from build123d import *

# Parameters (mm, degrees)
CUT_EXTRUDE1_DEPTH     = 5
CUT_EXTRUDE3_DEPTH     = 45
SKETCH8_R              = 40
CUT_EXTRUDE4_DEPTH     = 32
FILLET1_R              = 7
CUT_REVOLVE1_START     = 17
CUT_REVOLVE1_DEPTH     = 30.5
SKETCH18_W             = 13
SKETCH18_H             = 8
CUT_EXTRUDE13_DEPTH    = 5
SKETCH20_W             = 84
SKETCH20_H             = 7
CUT_EXTRUDE15_DEPTH    = 5
SKETCH19_R             = 1.5
CUT_EXTRUDE14_DEPTH    = 12
FILLET3_R              = 4
SKETCH21_W             = 16
SKETCH21_H             = 5
CUT_EXTRUDE16_DEPTH    = 5
CIRPATTERN1_COUNT      = 4
SKETCH22_W             = 5
SKETCH22_H             = 12
BOSS_EXTRUDE1_DEPTH    = 1.5
SKETCH23_W             = 5
SKETCH23_H             = 4.4
SKETCH23_H_2           = 4
BOSS_EXTRUDE2_DEPTH    = 17
SKETCH24_W             = 2
SKETCH24_H             = 3
BOSS_EXTRUDE3_DEPTH    = 2
CIRPATTERN2_COUNT      = 5
CUT_REVOLVE2_START     = 17
CUT_REVOLVE2_DEPTH     = 30.5
SKETCH29_W             = 16.2
SKETCH29_H             = 11.2
SKETCH29_W_2           = 13
SKETCH29_H_2           = 8
BOSS_EXTRUDE4_DEPTH    = 20
CUT_EXTRUDE18_DEPTH    = 12
SKETCH34_R             = 2.3
BOSS_EXTRUDE5_DEPTH    = 3.5
BOSS_EXTRUDE6_START    = 3.5
SKETCH35_R             = 2.3
BOSS_EXTRUDE6_DEPTH    = 3.5
SKETCH36_W             = 2
SKETCH36_H             = 2
BOSS_EXTRUDE7_DEPTH    = 5
SKETCH37_W             = 2
SKETCH37_H             = 2
BOSS_EXTRUDE8_DEPTH    = 12.5
SKETCH40_W             = 2
SKETCH40_H             = 2
BOSS_EXTRUDE9_DEPTH    = 5
INTERSECT7_START       = -43
INTERSECT7_OUTLINE_W   = 16.2
INTERSECT7_OUTLINE_H   = 20
INTERSECT7_OUTLINE_R   = 2.3
INTERSECT7_DEPTH       = 86
INTERSECT7_START_2     = -35.6
INTERSECT7_2_OUTLINE_W = 16.2
INTERSECT7_2_OUTLINE_H = 20
INTERSECT7_2_OUTLINE_R = 2.3
INTERSECT7_2_DEPTH     = 37.6


with BuildPart() as part:
    # Sketch1 → Revolve1 (revolve)
    with BuildSketch(Plane.XY, mode=Mode.PRIVATE) as revolve1_sk:
        with BuildLine():
            Line((37, 55), (0, 55))
            Line((0, 55), (0, 11.5))
            Line((0, 11.5), (22.5, 11.5))
            Line((22.5, 11.5), (22.5, 0))
            Line((22.5, 0), (25, 0))
            Line((25, 0), (25, 11.5))
            Line((25, 11.5), (42, 11.5))
            Line((42, 11.5), (42, 50))
            ThreePointArc((42, 50), (40.535533906, 53.535533906), (37, 55))
        make_face()
    revolve(revolve1_sk.sketch.rotate(Axis((0, 2, 0), (0, 1, 0)), 90), axis=Axis((0, 2, 0), (0, 1, 0)))

    # Sketch5 → Cut-Extrude1 (cut)
    with BuildSketch(Plane(origin=(0, 55, 0), x_dir=(1, 0, 0), z_dir=(0, 1, 0))):
        with BuildLine():
            Line((-42, 0), (-40, 0))
            Line((-40, 0), (40, 0))
            Line((40, 0), (42, 0))
            ThreePointArc((42, 0), (0, 42), (-42, 0))
        make_face()
    extrude(amount=-CUT_EXTRUDE1_DEPTH, mode=Mode.SUBTRACT)

    # Sketch7 → Cut-Extrude3 (cut)
    with BuildSketch(Plane.XZ.offset(-11.5)):
        with BuildLine():
            Line((21, 0), (-21, 0))
            ThreePointArc((-21, 0), (-18.277714988, -10.340461055), (-10.816653826, -18))
            Line((-10.816653826, -18), (10.816653826, -18))
            ThreePointArc((10.816653826, -18), (18.277714988, -10.340461055), (21, 0))
        make_face()
    extrude(amount=-CUT_EXTRUDE3_DEPTH, mode=Mode.SUBTRACT)

    # Sketch8 → Cut-Extrude4 (cut)
    with BuildSketch(Plane(origin=(0, 47.5, 0), x_dir=(1, 0, 0), z_dir=(0, 1, 0))):
        with Locations(Location((0, 0, 0), (0, 0, 270))):
            Circle(SKETCH8_R)
        with BuildLine():
            Line((22.912878475, -2), (-22.981606036, -2))
            ThreePointArc((-22.981606036, -2), (-20.067855169, 10.855581536), (-10.573881727, 20))
            Line((-10.573881727, 20), (10.505154166, 20))
            ThreePointArc((10.505154166, 20), (19.999127608, 10.855581536), (22.912878475, -2))
        make_face(mode=Mode.SUBTRACT)
    extrude(amount=-CUT_EXTRUDE4_DEPTH, mode=Mode.SUBTRACT)

    # Fillet1
    fillet1_edges = [part.edges().sort_by_distance(p)[0] for p in [
        (-21, 30.75, 0),
        (21, 30.75, 0),
    ]]
    fillet(fillet1_edges, radius=FILLET1_R)

    # Cut-Revolve1: read off the stored shape, not the designer's step
    # Cut-Revolve1 outline → Cut-Revolve1 (cut)
    with BuildSketch(Plane(origin=(0, 0, 0), x_dir=(1, 0, 0), z_dir=(0, 1, 0)).offset(CUT_REVOLVE1_START)):
        with BuildLine():
            Line((-34.641016151, -20), (-36.373066959, -21))
            ThreePointArc((-36.373066959, -21), (0, -42), (36.373066959, -21))
            Line((36.373066959, -21), (34.641016151, -20))
            ThreePointArc((34.641016151, -20), (0, -40), (-34.641016151, -20))
        make_face()
    extrude(amount=CUT_REVOLVE1_DEPTH, mode=Mode.SUBTRACT)

    # Sketch18 → Cut-Extrude13 (cut)
    with BuildSketch(Plane(origin=(0, 50, 0), x_dir=(1, 0, 0), z_dir=(0, 1, 0))):
        with Locations((0, 30)):
            Rectangle(SKETCH18_W, SKETCH18_H)
    extrude(amount=-CUT_EXTRUDE13_DEPTH, mode=Mode.SUBTRACT)

    # Sketch20 → Cut-Extrude15 (cut)
    with BuildSketch(Plane(origin=(0, 55, 0), x_dir=(1, 0, 0), z_dir=(0, 1, 0))):
        with Locations((0, -3.5)):
            Rectangle(SKETCH20_W, SKETCH20_H)
    extrude(amount=-CUT_EXTRUDE15_DEPTH, mode=Mode.SUBTRACT)

    # Sketch19 → Cut-Extrude14 (cut)
    with BuildSketch(Plane(origin=(0, 0, 7), x_dir=(-1, 0, 0), z_dir=(0, 0, -1))):
        with Locations((0, 52.5)):
            Circle(SKETCH19_R)
        with Locations((-29.412558482, 52.5)):
            Circle(SKETCH19_R)
        with Locations((29.412558482, 52.5)):
            Circle(SKETCH19_R)
    extrude(amount=-CUT_EXTRUDE14_DEPTH, mode=Mode.SUBTRACT)

    # Fillet3
    fillet3_edges = [part.edges().sort_by_distance(p)[0] for p in [
        (0, 11.5, 42),
    ]]
    fillet(fillet3_edges, radius=FILLET3_R)

    # Sketch21 → Cut-Extrude16 (cut)
    with BuildSketch(Plane(origin=(0, 15.5, 0), x_dir=(1, 0, 0), z_dir=(0, 1, 0))):
        with Locations((0, -29.5)):
            Rectangle(SKETCH21_W, SKETCH21_H)
    cut_extrude16 = extrude(amount=-CUT_EXTRUDE16_DEPTH, mode=Mode.SUBTRACT)

    # CirPattern1: Cut-Extrude16 ×4 about axis
    cirpattern1_axis = Axis((0, 0, 0), (0, 1, 0))
    for i in range(1, CIRPATTERN1_COUNT):
        add(cut_extrude16.rotate(cirpattern1_axis, i * 360 / CIRPATTERN1_COUNT), mode=Mode.SUBTRACT)

    # Sketch22 → Boss-Extrude1 (add)
    with BuildSketch(Plane(origin=(0, 15.5, 0), x_dir=(1, 0, 0), z_dir=(0, 1, 0))):
        with Locations((35.5, -4)):
            Rectangle(SKETCH22_W, SKETCH22_H)
    extrude(amount=BOSS_EXTRUDE1_DEPTH)

    # Sketch23 → Boss-Extrude2 (add)
    with BuildSketch(Plane(origin=(0, 17, 0), x_dir=(1, 0, 0), z_dir=(0, 1, 0))):
        with Locations((35.5, -0.2)):
            Rectangle(SKETCH23_W, SKETCH23_H)
        with Locations((35.5, -8)):
            Rectangle(SKETCH23_W, SKETCH23_H_2)
    extrude(amount=BOSS_EXTRUDE2_DEPTH)

    # Sketch24 → Boss-Extrude3 (add)
    with BuildSketch(Plane.XZ):
        with Locations((0, -22.5)):
            Rectangle(SKETCH24_W, SKETCH24_H)
    boss_extrude3 = extrude(amount=-BOSS_EXTRUDE3_DEPTH)

    # CirPattern2: Boss-Extrude3 ×5 about axis
    cirpattern2_axis = Axis((0, 0, 0), (0, 1, 0))
    for i in range(1, CIRPATTERN2_COUNT):
        add(boss_extrude3.rotate(cirpattern2_axis, i * 360 / CIRPATTERN2_COUNT))

    # Cut-Revolve2: read off the stored shape, not the designer's step
    # Cut-Revolve2 outline → Cut-Revolve2 (cut)
    with BuildSketch(Plane(origin=(0, 0, 0), x_dir=(1, 0, 0), z_dir=(0, 1, 0)).offset(CUT_REVOLVE2_START)):
        with BuildLine():
            ThreePointArc((-30.641777725, 25.711504387), (0, 40), (30.641777725, 25.711504387))
            Line((30.641777725, 25.711504387), (32.173866611, 26.997079607))
            ThreePointArc((32.173866611, 26.997079607), (0, 42), (-32.173866611, 26.997079607))
            Line((-32.173866611, 26.997079607), (-30.641777725, 25.711504387))
        make_face()
    extrude(amount=CUT_REVOLVE2_DEPTH, mode=Mode.SUBTRACT)

    # Sketch29 → Boss-Extrude4 (add)
    with BuildSketch(Plane.XZ.offset(-47.5)):
        with Locations((0, -30)):
            Rectangle(SKETCH29_W, SKETCH29_H)
        with Locations((0, -30)):
            Rectangle(SKETCH29_W_2, SKETCH29_H_2, mode=Mode.SUBTRACT)
    extrude(amount=BOSS_EXTRUDE4_DEPTH)

    # Sketch32 → Cut-Extrude18 (cut)
    with BuildSketch(Plane(origin=(0, 0, -35.6), x_dir=(-1, 0, 0), z_dir=(0, 0, -1))):
        with BuildLine():
            Line((-4.55, 40.24987133), (-4.55, 41.2))
            ThreePointArc((-4.55, 41.2), (-4.258194078, 41.946205288), (-3.537595761, 42.296506718))
            ThreePointArc((-3.537595761, 42.296506718), (0, 45.55), (3.537595761, 42.296506718))
            ThreePointArc((3.537595761, 42.296506718), (4.258194078, 41.946205288), (4.55, 41.2))
            Line((4.55, 41.2), (4.55, 40.675870248))
            ThreePointArc((4.55, 40.675870248), (4.010824187, 37.38705417), (2.4497454, 34.442558497))
            ThreePointArc((2.4497454, 34.442558497), (1.613339464, 32.35352404), (1.966232927, 30.131114075))
            ThreePointArc((1.966232927, 30.131114075), (1.891748397, 29.932488662), (1.693122984, 30.006973192))
            ThreePointArc((1.693122984, 30.006973192), (1.315208372, 32.386958334), (2.210917864, 34.624111266))
            ThreePointArc((2.210917864, 34.624111266), (3.726528337, 37.48284493), (4.25, 40.675870248))
            Line((4.25, 40.675870248), (4.25, 41.2))
            ThreePointArc((4.25, 41.2), (4.015685425, 41.765685425), (3.45, 42))
            Line((3.45, 42), (3.25, 42))
            ThreePointArc((3.25, 42), (0, 45.25), (-3.25, 42))
            Line((-3.25, 42), (-3.45, 42))
            ThreePointArc((-3.45, 42), (-4.015685425, 41.765685425), (-4.25, 41.2))
            Line((-4.25, 41.2), (-4.25, 40.24987133))
            ThreePointArc((-4.25, 40.24987133), (-3.782078371, 37.22671372), (-2.422103613, 34.486476277))
            ThreePointArc((-2.422103613, 34.486476277), (-1.704952932, 32.326507722), (-2.304950317, 30.131109718))
            ThreePointArc((-2.304950317, 30.131109718), (-2.51173821, 30.0837941), (-2.559053827, 30.290581992))
            ThreePointArc((-2.559053827, 30.290581992), (-2.00484446, 32.318441057), (-2.667266721, 34.313574426))
            ThreePointArc((-2.667266721, 34.313574426), (-4.068040722, 37.136018992), (-4.55, 40.24987133))
        make_face()
    extrude(amount=-CUT_EXTRUDE18_DEPTH, mode=Mode.SUBTRACT)

    # Sketch34 → Boss-Extrude5 (add)
    with BuildSketch(Plane.XY.offset(-34)):
        with Locations(Location((0, 42, 0), (0, 0, 180))):
            Circle(SKETCH34_R)
    extrude(amount=BOSS_EXTRUDE5_DEPTH)

    # Sketch35 → Boss-Extrude6 (add)
    with BuildSketch(Plane(origin=(0, 0, -26), x_dir=(-1, 0, 0), z_dir=(0, 0, -1)).offset(BOSS_EXTRUDE6_START)):
        with Locations((0, 42)):
            Circle(SKETCH35_R)
    extrude(amount=-BOSS_EXTRUDE6_DEPTH)

    # Sketch36 → Boss-Extrude7 (add)
    with BuildSketch(Plane(origin=(0, 0, -35.6), x_dir=(-1, 0, 0), z_dir=(0, 0, -1))):
        with Locations((-6.159647943, 37.918102195)):
            Rectangle(SKETCH36_W, SKETCH36_H)
    extrude(amount=BOSS_EXTRUDE7_DEPTH)

    # Sketch37 → Boss-Extrude8 (add)
    with BuildSketch(Plane.ZY.offset(-5.159647943)):
        with Locations((-39.597351245, 37.918102195)):
            Rectangle(SKETCH37_W, SKETCH37_H)
    extrude(amount=BOSS_EXTRUDE8_DEPTH)

    # Sketch40 → Boss-Extrude9 (add)
    with BuildSketch(Plane(origin=(0, 0, -35.6), x_dir=(-1, 0, 0), z_dir=(0, 0, -1))):
        with Locations((6.340352057, 37.918102195)):
            Rectangle(SKETCH40_W, SKETCH40_H)
    extrude(amount=BOSS_EXTRUDE9_DEPTH)

    # Intersect7: read off the stored shape, not the designer's step
    # Intersect7 outline → Intersect7 (cut)
    # profile 1 of 2: a face of its own
    with BuildSketch(Plane.XY.offset(INTERSECT7_START)):
        Polygon((44, 55), (-44, 55), (-44, 11.5), (-27, 11.5), (-27, 0), (27, 0), (27, 11.5), (44, 11.5), align=None)
        with Locations((0, 37.5)):
            Rectangle(INTERSECT7_OUTLINE_W, INTERSECT7_OUTLINE_H, mode=Mode.SUBTRACT)
    # profile 2 of 2: a face of its own
    with BuildSketch(Plane.XY.offset(INTERSECT7_START)):
        with Locations((0, 42)):
            Circle(INTERSECT7_OUTLINE_R)
    extrude(amount=INTERSECT7_DEPTH, mode=Mode.SUBTRACT)

    # Intersect7 2 outline → Intersect7 2 (cut)
    with BuildSketch(Plane.XY.offset(INTERSECT7_START_2)):
        with Locations((0, 37.5)):
            Rectangle(INTERSECT7_2_OUTLINE_W, INTERSECT7_2_OUTLINE_H)
        with Locations((0, 42)):
            Circle(INTERSECT7_2_OUTLINE_R, mode=Mode.SUBTRACT)
    extrude(amount=INTERSECT7_2_DEPTH, mode=Mode.SUBTRACT)


solid = part.part
Source: CAD feature listing. Evaluate the final solid. Frame: model axes, mm. A direction names the side the tool comes from. Round coordinates to 2 decimals unless told otherwise and drop trailing zeros. Loops run counter-clockwise (first coordinate to the right, second up) from the corner with the lowest first, then second, coordinate; pieces in that order, holes last. Notation, with made-up numbers: M 75,-24 L 125,-24 A18 cw 125,6 Z; hole C 17,33 d8. An arc over 180 degrees is marked long. Answer as CSV lines item,"result".
Q1. Cut plane C-C (x = -3). Return the cut outline in (y, z), plus the area to 3 significant figures.
Verdict:
outline,"M 36.92,-40.6 L 38.92,-40.6 L 38.92,-38.6 L 36.92,-38.6 Z"
area,"4.00 mm^2"
Q2. Line query: line 1 along X through (y, z) = (38, -36.4); line 2 along Z through (x, y) = (-1.75, 38.55). Output: solid intervals per line, ascending.
Verdict:
line 1,"x = -7.34 to -5.34, 5.16 to 7.16"
line 2,"z = -40.6 to -38.6"
Q3. Contact query for a flat-ended pin moving along its axis: pin 1 (1 mm diameter, centred on x = -1.5, y = 37.5, fed in from +Z). Output: stop coordinate, or through.
Verdict:
pin 1,"stops at z = -38.6"
Q4. Reachability of faces 5 (the face through (-5.34, 38, -37)), 6 (the face through (0, 38.918, -39)) from +Z, -Z, +X, -X, +Y, -Y: full face, straight path, thin tool, end or side. Return the list, or none.
Verdict:
face 5,"+Z, +Y, -Y"
face 6,"+Z, -Z, +X, -X, +Y"
Q5. Cut plane A-A (z = -36.4). Return the cut outline in (x, y).
Verdict:
outline,"M -7.34,36.92 L -5.34,36.92 L -5.34,38.92 L -7.34,38.92 Z; M 5.16,36.92 L 7.16,36.92 L 7.16,38.92 L 5.16,38.92 Z"
Q6. Pull-direction query (X, two-part tool) for faces 1 (the face through (-7.34, 38, -38)), 2 (the face through (0, 38, -38.597)), 3 (the face through (7.16, 38, -38)), 4 (the face through (-6, 38, -35.6)); classes: +X half, -X half, draft (parallel to the pull), parting line (faces both ways), or undercut.
Verdict:
face 1,"-X half"
face 2,"undercut"
face 3,"+X half"
face 4,"draft"
